Part print with two shaded views. Sizes in mm from the minimum x, y, z corner. Round coordinates to 2 decimals unless told otherwise and drop trailing zeros. Loops run counter-clockwise (first coordinate to the right, second up) from the corner with the lowest first, then second, coordinate; pieces in that order, holes last. Notation, with made-up numbers: (-19.5, 58.25) -> (-11.5, 58.25) arc R25 cw to (-11.5, 92.25) -> close; hole circle Ø2 at (70, 18). An arc over 180 degrees is marked (long way). Use a Markdown table: item, result. Add a question column.
Item 1: Flat gauge pins, fed straight in: pin 1 (6 mm diameter, centred on y = 11, z = 70.5, fed in from +X); pin 2 (4 mm diameter, centred on x = 10, z = 72.5, fed in from +Y); pin 3 (2.5 mm diameter, centred on x = 6.35, y = 6.35, fed in from -Z); pin 4 (4.5 mm diameter, centred on x = 6.35, z = 20.25, fed in from -Y). Where does each tip first touch, or does it go through?
Item 2: Cut at C-C, the plane x = 1.5. List the corners of the cut face in (y, z).
Item 3: Probe line 1 (X direction, y = 6.5, z = 20.25); line 2 (Z direction, x = 7.25, y = 5) (1 decimal); line 3 (Z direction, x = 8, y = 10.5). List the from-to ranges inside material, lowest first. Write a range as [from, to].
Item 4: Cut at B-B, the plane z = 61. List the corners of the cut face in (x, y), plus the area to 3 significant figures.
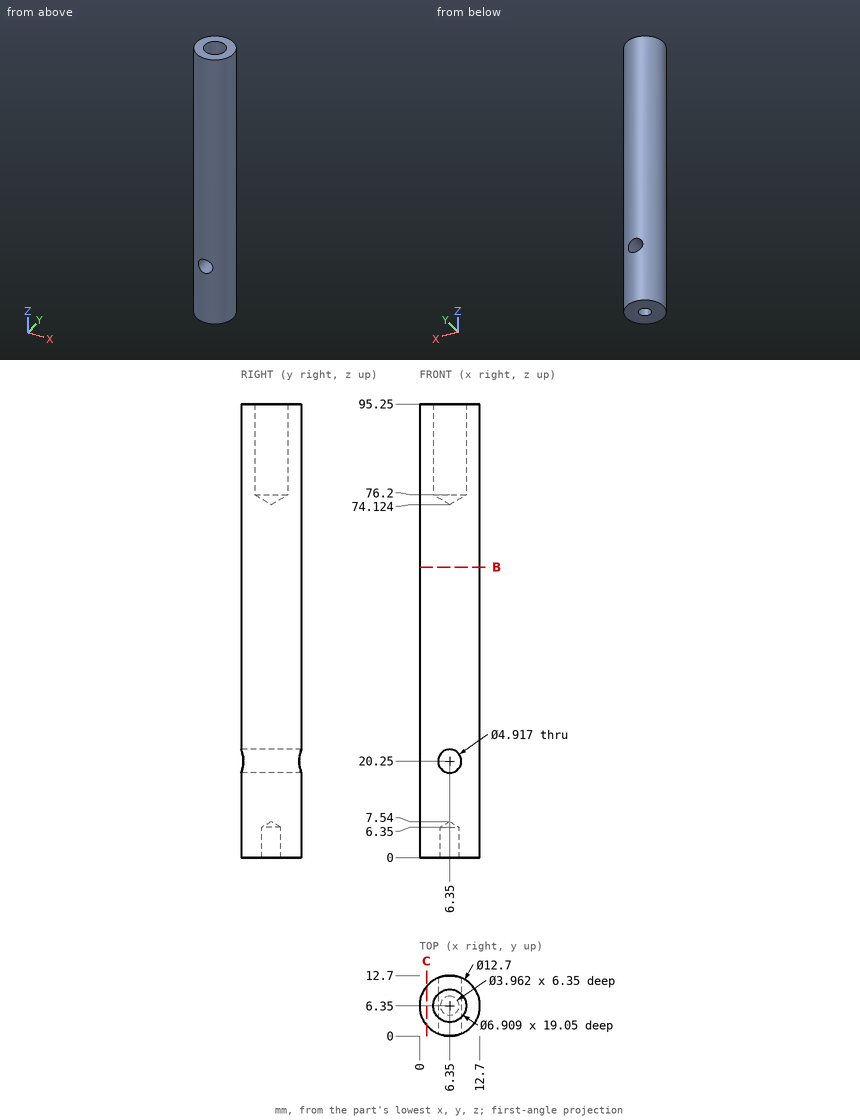
A:
| question | item | result |
|---|---|---|
| 1 | pin 1 | stops at x = 12.48 |
| 1 | pin 2 | stops at y = 12.48 |
| 1 | pin 3 | stops at z = 6.79 |
| 1 | pin 4 | passes through |
| 2 | outline | (2.25, 0) -> (10.45, 0) -> (10.45, 95.25) -> (2.25, 95.25) -> close |
| 3 | line 1 | x = [0, 3.89], [8.81, 12.7] |
| 3 | line 2 | z = [6.6, 18], [22.5, 75.1] |
| 3 | line 3 | z = [0, 18.43], [22.07, 95.25] |
| 4 | outline | circle Ø12.7 at (6.35, 6.35) |
| 4 | area | 127 mm^2 |
